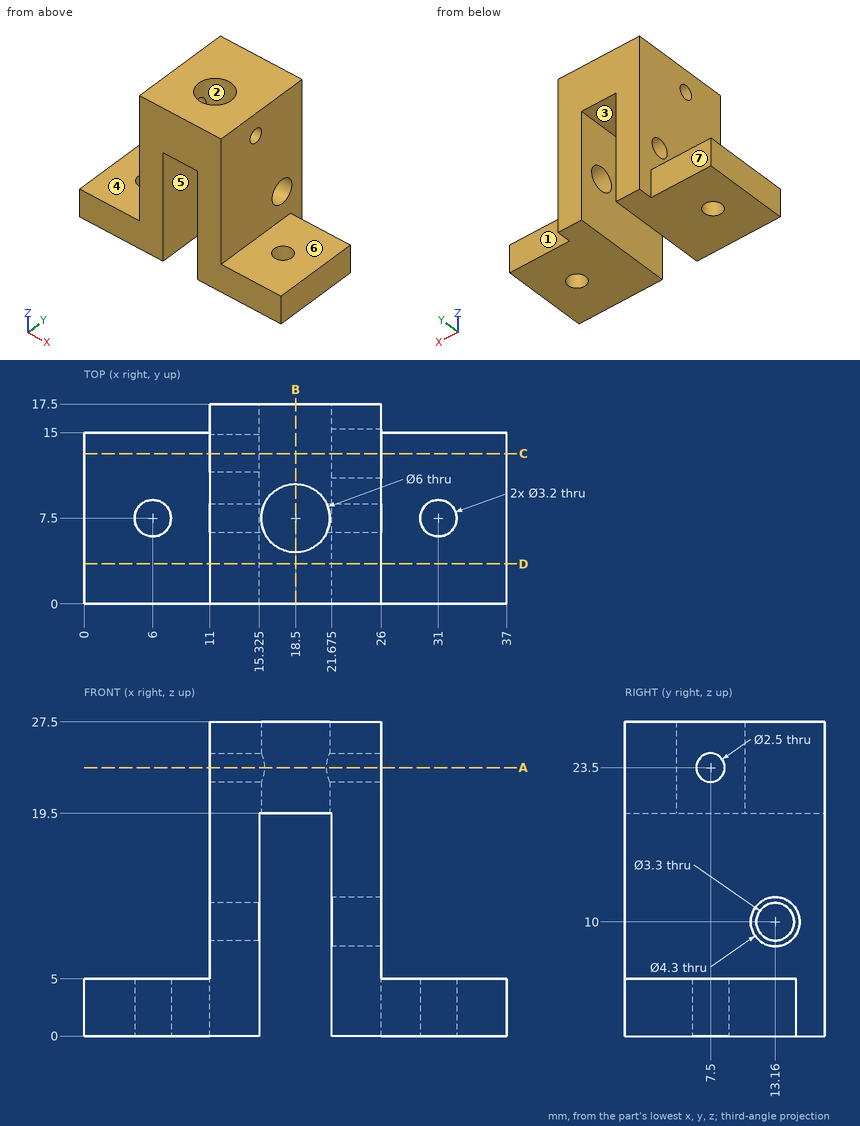
Print and shaded views of the part. All mm, measured from the part's lowest x, y and z. A direction names the side the tool comes from. Give positions to 0.01 mm unless a question says otherwise; leave off trailing zeros. Loops run counter-clockwise (first coordinate to the right, second up) from the corner with the lowest first, then second, coordinate; pieces in that order, holes last. Notation, with made-up numbers: (15.25, 62) -> (72.25, 62) arc R20 ccw to (72.25, 85) -> close; hole circle Ø1 at (46.25, 81.5). An arc over 180 degrees is marked (long way). Answer in a Markdown table with one row per item.
Item 1: Probe line 1 along X through (y, z) = (14.75, 11.5) (3 decimals); line 2 along X through (y, z) = (2.5, 2) (3 decimals); line 3 along Z through (x, y) = (13.85, 7.5). List the from-to ranges inside material, lowest first. Write a range as [from, to].
Findings below:
| item | result |
|---|---|
| line 1 | x = [11, 15.325], [21.675, 26] |
| line 2 | x = [0, 15.325], [21.675, 37] |
| line 3 | z = [0, 22.25], [24.75, 27.5] |
Item 2: Slice it at A-A on z = 23.5. Write the cut outline in (x, y), plus the area to 3 significant figures.
Findings below:
| item | result |
|---|---|
| outline | (11, 0) -> (26, 0) -> (26, 6.25) -> (21.23, 6.25) arc R3 cw to (15.77, 6.25) -> (11, 6.25) -> close; (11, 8.75) -> (15.77, 8.75) arc R3 cw to (21.23, 8.75) -> (26, 8.75) -> (26, 17.5) -> (11, 17.5) -> close |
| area | 211 mm² |
Item 3: Flat gauge pins, fed straight in: P1, Ø3.5, axis at y = 13.16, z = 10, coming from the -X side; P2, Ø1.5, axis at x = 32.5, z = 1.5, coming from the +Y side; P3, Ø3, axis at x = 31, y = 7.5, coming from the -Z side; P4, Ø5.5, axis at x = 34, y = 8.5, coming from the +Z side. Where does each tip first touch, or does it go through?
Findings below:
| item | result |
|---|---|
| P1 | stops at x = 11 |
| P2 | stops at y = 15 |
| P3 | passes through |
| P4 | stops at z = 5 |
Item 4: Slice it at D-D on y = 3.5. Write the cut outline in (x, z) (3 decimals), plus the area to 3 significant figures.
Findings below:
| item | result |
|---|---|
| outline | (0, 0) -> (15.325, 0) -> (15.325, 19.5) -> (21.675, 19.5) -> (21.675, 0) -> (37, 0) -> (37, 5) -> (26, 5) -> (26, 27.5) -> (11, 27.5) -> (11, 5) -> (0, 5) -> close |
| area | 399 mm² |
Item 5: Slice it at B-B on x = 18.5. Write the cut outline in (y, z).
Findings below:
| item | result |
|---|---|
| outline | (0, 19.5) -> (4.5, 19.5) -> (4.5, 27.5) -> (0, 27.5) -> close; (10.5, 19.5) -> (17.5, 19.5) -> (17.5, 27.5) -> (10.5, 27.5) -> close |
Item 6: Mould opens along Y. For the marked faces 1, 2 and 3 say: pulls with the +Y half, pulls with the -Y half, needs draft (parallel to the pull), parting line crosses it, or undercut.
Findings below:
| item | result |
|---|---|
| face 1 | pulls with the +Y half |
| face 2 | undercut |
| face 3 | needs draft |
Item 7: Tool access for the marked faces 4, 5, 6 and 7: list every direction of +Z, -Z, +X, -X, +Y, -Y with a clear straight run to the whole face (end or side of a thin tool).
Findings below:
| item | result |
|---|---|
| face 4 | +Z, -X, +Y, -Y |
| face 5 | -Z, +Y, -Y |
| face 6 | +Z, +X, +Y, -Y |
| face 7 | +Z, -Z, -X, +Y |
Item 8: Slice it at C-C on y = 13.16. Write the cut outline in (x, z) (3 decimals), plus the area to 3 significant figures.
Findings below:
| item | result |
|---|---|
| outline | (0, 0) -> (15.325, 0) -> (15.325, 8.35) -> (11, 8.35) -> (11, 5) -> (0, 5) -> close; (11, 11.65) -> (15.325, 11.65) -> (15.325, 19.5) -> (21.675, 19.5) -> (21.675, 12.15) -> (26, 12.15) -> (26, 27.5) -> (11, 27.5) -> close; (21.675, 0) -> (37, 0) -> (37, 5) -> (26, 5) -> (26, 7.85) -> (21.675, 7.85) -> close |
| area | 366 mm² |
